Autodesk Inventor part; units mm, degrees
ref_plane "YZ Plane" through (0, 0, 0) normal (1, 0, 0) x (0, 1, 0)
ref_plane "XZ Plane" through (0, 0, 0) normal (0, 1, 0) x (-1, 0, 0)
ref_plane "XY Plane" through (0, 0, 0) normal (0, 0, 1) x (1, 0, 0)
sketch "Esquisse1" plane through (0, 0, 0) normal (1, 0, 0) x (0, 1, 0)
  line L0 (0, 0) -> (0, -23.6667)
  line L1 (9.5, 0) -> (7.5, 0)
  line L2 (7.5, 0) -> (7.5, -43)
  line L3 (11, -35) -> (11, -41)
  line L4 (7.5, -43) -> (0, -43)
  line L5 (11, -46) -> (0, -46)
  line L6 (0, -43) -> (0, -46)
  line L7 (11, -46) -> (12, -41)
  line L8 (12, -41) -> (11, -41)
  line L9 (11, -35) -> (9.5, -35)
  line L10 (9.5, 0) -> (9.5, -35)
  dimension "d1" = 15
  dimension "d2" = 43
  dimension "d3" = 3
  dimension "d8" = 22
  dimension "d9" = 1
  dimension "d10" = 5
  dimension "d11" = 19
  dimension "d12" = 6
revolve "Révolution1" add sketch "Esquisse1" angle 360 about axis through (0, 0, 0) along (0, 0, -1)
chamfer "Chanfrein1" distance 1 angle 45 1 edges at (0, -7.5, -43)
sketch "Esquisse2" plane through (0, 0, -46) normal (0, 0, -1) x (-1, 0, 0)
  line L0 (5.4848, 9.5) -> (10.9697, 0)
  line L1 (10.9697, 0) -> (5.4848, -9.5)
  line L2 (5.4848, -9.5) -> (-5.4848, -9.5)
  line L3 (-5.4848, -9.5) -> (-10.9697, 0)
  line L4 (-10.9697, 0) -> (-5.4848, 9.5)
  line L5 (-5.4848, 9.5) -> (5.4848, 9.5)
  circle A0 centre (0, 0) radius 12
  circle A1 centre (0, 0) radius 11
  dimension "d13" = 19
extrude "Extrusion1" cut sketch "Esquisse2" against normal blind 4 contours A0 | A1
thread "Filetage1"
chamfer "Chanfrein2" distance 1 angle 45 1 edges at (0, -11, -35)
properties part number "piston_corps"
Could you check a few things on this model? Use its own coordinates, in mm. A direction names the side the tool comes from. Give positions to 0.01 mm unless a question says otherwise; leave off trailing zeros. Loops run counter-clockwise (first coordinate to the right, second up) from the corner with the lowest first, then second, coordinate; pieces in that order, holes last. Notation, with made-up numbers: (56, 56.5) -> (71, 56.5) arc R24 ccw to (71, 69.5) -> close; hole circle Ø2 at (-27, -37). An arc over 180 degrees is marked (long way). Answer as CSV lines item,"result". Start each with the question number.
(1) If we section it at B-B on z = -5.5: Write out the boundary of the cut face in (x, y).
(2) Which directions (+Z, -Z, +X, -X, +Y, -Y) give clear straight access to the entire face, cutting with the end or side of a thin tool? Please do faces 4 (the flat face through (0, 10, -42)), 5 (the flat face through (0, -9.5, -44)), 6 (the cylindrical face through (-10.74, -2.38, -38.53)).
(3) We'd pull the mould along X, two halves only. Please class faces 1 (the flat face through (8.2, -4.8, -44)), 2 (the flat face through (-8.266, -4.683, -44.028)), 3 (the flat face through (0, 0, -43)): released by +X, released by -X, zero draft, split by the parting line, or undercut.
(4) I'm going to push flat-ended pins straight in: pin 1 Ø4.5 at (x, z) = (0, -44) entering from -Y; pin 2 Ø3 at (y, z) = (-1.5, -34.5) entering from +X; pin 3 Ø4 at (x, z) = (2.5, -32.5) entering from -Y. Where does each tip first touch, or does it pass through?
(5) If we section it at C-C on z = -39.5: Write out the boundary of the cut face in (x, y).
(6) I need wall thicknesses on probe 1 along Y at (x, z) = (0.25, -4.5); probe 2 along Z at (x, y) = (-6, -2). Which ranges of each line are inside material? Lowest first, please.
(7) If we section it at A-A on x = 0: Write out the boundary of the cut face in (y, z).
Computed:
1,outline,"circle Ø19 at (0, 0); hole circle Ø15 at (0, 0)"
2,face 4,"-Z"
2,face 5,"-Z, +X, -X, -Y"
2,face 6,"+Z"
3,face 1,"released by +X"
3,face 2,"released by -X"
3,face 3,"undercut"
4,pin 1,"stops at y = -11.85"
4,pin 2,"stops at x = 10.91"
4,pin 3,"stops at y = -9.49"
5,outline,"circle Ø22 at (0, 0); hole circle Ø15 at (0, 0)"
6,probe 1,"y = -9.5 to -7.5, 7.5 to 9.5"
6,probe 2,"z = -46 to -43"
7,outline,"(-12, -41) -> (-11.8, -42) -> (-9.5, -42) -> (-9.5, -46) -> (9.5, -46) -> (9.5, -42) -> (11.8, -42) -> (12, -41) -> (11, -41) -> (11, -36) -> (10, -35) -> (9.5, -35) -> (9.5, 0) -> (7.5, 0) -> (7.5, -42) -> (6.5, -43) -> (-6.5, -43) -> (-7.5, -42) -> (-7.5, 0) -> (-9.5, 0) -> (-9.5, -35) -> (-10, -35) -> (-11, -36) -> (-11, -41) -> close"
